Geometry: final body of the model. Coordinates: model frame, mm. A direction names the side the tool comes from. Give positions to 0.01 mm unless a question says otherwise; leave off trailing zeros. Write each loop counter-clockwise with the first axis right and the second up, starting at its lowest first coordinate (ties: lowest second). Pieces come first, ordered by that corner, then holes. Notation, with made-up numbers: M -1,2.5 L 51,2.5 A26 cw 51,23.5 Z; hole C 56.5,47.25 d7. An arc over 180 degrees is marked long. Use a Markdown table: item, result. Add a question column.
1) Section C-C on y = 14. Return the cut outline in (x, z).
2) Set-up query: faces 4 (the flat face through (0, 34.2, 0)), 5 (the cylindrical face through (-7.33, 29.72, 0.69)), 6 (the cylindrical face through (0.07, 1.48, -6.5)). Return all of +Z, -Z, +X, -X, +Y, -Y with unobstructed straight access to the full face (end or side cutting, diameter ignored); none if empty.
3) Draft query along Z for faces 1 (the cylindrical face through (-13.67, 13.41, -3.03)), 2 (the flat face through (-9, 3, 0)), 3 (the flat face through (-2, 31.2, 0)). Return one class per face: +Z half, -Z half, draft (parallel to the pull), parting line (faces both ways), or undercut.
4) Line query: line 1 (X direction, y = 2, z = 0); line 2 (Y direction, x = -3.75, z = 5.75); line 3 (Z direction, x = -0.25, y = 4.5). Output: solid intervals per line, ascending.
5) Pin query (flat end, axial travel): pin 1 (2.5 mm diameter, centred on x = -0.5, z = 5.5, fed in from +Y); pin 2 (0.9 mm diameter, centred on x = 9.5, z = -0.5, fed in from -Y); pin 3 (6 mm diameter, centred on x = 3, z = -1.5, fed in from +Y); pin 4 (1.5 mm diameter, centred on y = 15.5, z = -7.5, fed in from -X). Return the tip coordinate at first contact, or that it passes through.
```python
from build123d import *

# Parameters (mm, degrees)
SKIZZE1_R                       = 14
AUFSATZ_LINEAR_AUSTRAGEN1_DEPTH = 31.2
FASE1_SIZE                      = 4
FASE1_SIZE2                     = 6
SKIZZE2_R                       = 1.033731655
AUFSATZ_LINEAR_AUSTRAGEN2_DEPTH = 3
SKIZZE3_R                       = 1.5
SCHNITT_LINEAR_AUSTRAGEN1_DEPTH = 3
SKIZZE4_R                       = 3.1
AUFSATZ_LINEAR_AUSTRAGEN3_DEPTH = 3
SKIZZE5_R                       = 1.5
SCHNITT_LINEAR_AUSTRAGEN2_DEPTH = 3


with BuildPart() as part:
    # Skizze1 → Aufsatz-Linear austragen1 (new body)
    with BuildSketch(Plane(origin=(0, 0, 0), x_dir=(1, 0, 0), z_dir=(0, 1, 0))):
        with Locations(Location((0, 0, 0), (0, 0, 270))):
            Circle(SKIZZE1_R)
    extrude(amount=AUFSATZ_LINEAR_AUSTRAGEN1_DEPTH)

    # Fase1
    fase1_edges = [part.edges().sort_by_distance(p)[0] for p in [
        (0, 31.2, -14),
    ]]
    fase1_side = [part.faces().sort_by_distance(p)[0] for p in [
        (0, 15.6, -14),
    ]]
    chamfer(fase1_edges, length=FASE1_SIZE, length2=FASE1_SIZE2, reference=fase1_side[0])

    # Skizze2 → Aufsatz-Linear austragen2 (add)
    with BuildSketch(Plane(origin=(0, 31.2, 0), x_dir=(1, 0, 0), z_dir=(0, 1, 0))):
        with Locations(Location((0, 0, 0), (0, 0, 270))):
            Circle(SKIZZE2_R)
    extrude(amount=AUFSATZ_LINEAR_AUSTRAGEN2_DEPTH)

    # Skizze3 → Schnitt-Linear austragen1 (cut)
    with BuildSketch(Plane(origin=(0, 31.2, 0), x_dir=(1, 0, 0), z_dir=(0, 1, 0))):
        with Locations(Location((-6, 0, 0), (0, 0, 270))):
            Circle(SKIZZE3_R)
        with Locations(Location((0, 6, 0), (0, 0, 270))):
            Circle(SKIZZE3_R)
        with Locations(Location((6, 0, 0), (0, 0, 270))):
            Circle(SKIZZE3_R)
        with Locations(Location((0, -6, 0), (0, 0, 270))):
            Circle(SKIZZE3_R)
    extrude(amount=-SCHNITT_LINEAR_AUSTRAGEN1_DEPTH, mode=Mode.SUBTRACT)

    # Skizze4 → Aufsatz-Linear austragen3 (add)
    with BuildSketch(Plane.XZ):
        with Locations(Location((0, 0, 0), (0, 0, 270))):
            Circle(SKIZZE4_R)
    extrude(amount=AUFSATZ_LINEAR_AUSTRAGEN3_DEPTH)

    # Skizze5 → Schnitt-Linear austragen2 (cut)
    with BuildSketch(Plane.XZ):
        with Locations(Location((0, 8, 0), (0, 0, 270))):
            Circle(SKIZZE5_R)
        with Locations(Location((-9.5, 0, 0), (0, 0, 270))):
            Circle(SKIZZE5_R)
        with Locations(Location((9.5, 0, 0), (0, 0, 270))):
            Circle(SKIZZE5_R)
        with Locations(Location((0, -8, 0), (0, 0, 270))):
            Circle(SKIZZE5_R)
    extrude(amount=-SCHNITT_LINEAR_AUSTRAGEN2_DEPTH, mode=Mode.SUBTRACT)


solid = part.part
```
Found:
| question | item | result |
|---|---|---|
| 1 | outline | C 0,0 d28 |
| 2 | face 4 | +Z, -Z, +X, -X, +Y |
| 2 | face 5 | +Y |
| 2 | face 6 | -Y |
| 3 | face 1 | parting line |
| 3 | face 2 | undercut |
| 3 | face 3 | draft |
| 4 | line 1 | -14 to -11, -8 to 8, 11 to 14 |
| 4 | line 2 | 0 to 31.2 |
| 4 | line 3 | -14 to 14 |
| 5 | pin 1 | y = 31.2 |
| 5 | pin 2 | y = 3 |
| 5 | pin 3 | y = 34.2 |
| 5 | pin 4 | x = -12.27 |
